For this review, take the finished solid that the model builds, in its own axes (mm). Face numbers are marked on the shaded views. A direction names the side the tool comes from. Round coordinates to 2 decimals unless told otherwise and drop trailing zeros. Loops run counter-clockwise (first coordinate to the right, second up) from the corner with the lowest first, then second, coordinate; pieces in that order, holes last. Notation, with made-up numbers: (77, 63.25) -> (136, 63.25) arc R25 ccw to (136, 77.25) -> close; hole circle Ø9 at (-39.5, 86.25). An arc over 180 degrees is marked (long way). One line per question, with ' | ' between items. Start each with the question number.
1. For pin 1 Ø3 at (y, z) = (-17.5, -16.5) entering from +X; pin 2 Ø2 at (x, y) = (-32, -4.5) entering from -Z; pin 3 Ø2.5 at (x, y) = (-31, -20) entering from -Z, all flat-tipped, find the tip position at first contact; note any pin that passes through.
2. Consider section A-A (y = -23.5). Write out the cut boundary in (x, z), and give its area (3 significant figures).
3. Consider section B-B (x = -27.5). Count the separate pieces of the cut face and the enclosed holes in it, and give its area (3 significant figures).
4. Wall thickness on line 1 along Z through (x, y) = (-25, -9); line 2 along Z through (x, y) = (-19, -36); line 3 along X through (y, z) = (-17, 35): over which ranges is each line inside the solid? List them lowest first.
5. For the marked faces 1, 2 and 3, list the 3-axis set-ups (+Z, -Z, +X, -X, +Y, -Y) from which the entire face can be reached by the end or side of a thin tool; tool diameter is ignored.
6. Draft analysis for pull direction Z (two halves, no side actions). For the marked faces 4, 5 and 6, state which applies: pulls with the +Z half, pulls with the -Z half, needs draft (parallel to the pull), parting line crosses it, or undercut.
```python
from build123d import *

# Parameters (mm, degrees)
F1_DEPTH = 12.7
F2_DEPTH = 25.4
F3_R     = 5.08


with BuildPart() as f1:
    # F0 (on Front) → F1 (new body)
    with BuildSketch(Plane.XZ):
        Polygon((-29.3797869235, -7.2736367583), (-29.3797869235, -44.0696775913), (14.8325152695, -44.0696775913), (15.1177551597, -3.8507485297), (-5.1343315281, 28.666684404), (-5.1343315281, 42.6434762776), (9.1277007014, 42.6434762776), (3.1376483385, 52.341658622), (-34.2288762331, 52.341658622), (-34.2288762331, 46.6368459165), (-25.9568989277, 46.6368459165), (-39.0779674053, 25.529038161), (-39.0779674053, 16.6865773499), (-33.0879166722, 22.1061483026), (-23.674974218, 38.6501066387), (-17.3996798694, 24.958556518), (-17.3996798694, 9.8408022895), align=None)
    extrude(amount=F1_DEPTH)

    # F0 (on Front) + F1_face (on face) + F1_face1 (on face) → F2 (join)
    with BuildSketch(Plane.XZ):
        Polygon((-29.3797869235, -7.2736367583), (-29.3797869235, -44.0696775913), (14.8325152695, -44.0696775913), (15.1177551597, -3.8507485297), (-5.1343315281, 28.666684404), (-5.1343315281, 42.6434762776), (9.1277007014, 42.6434762776), (3.1376483385, 52.341658622), (-34.2288762331, 52.341658622), (-34.2288762331, 46.6368459165), (-25.9568989277, 46.6368459165), (-39.0779674053, 25.529038161), (-39.0779674053, 16.6865773499), (-33.0879166722, 22.1061483026), (-23.674974218, 38.6501066387), (-17.3996798694, 24.958556518), (-17.3996798694, 9.8408022895), align=None)
    with BuildSketch(Plane(origin=(-9.327897656, -12.7, -1.3317405801), x_dir=(1, 0, 0), z_dir=(0, -1, 0))):
        Polygon((18.4555983573, 43.9752168577), (12.4655459944, 53.6733992022), (-24.9009785771, 53.6733992022), (-24.9009785771, 47.9685864966), (-16.6290012717, 47.9685864966), (-29.7500697493, 26.8607787412), (-29.7500697493, 18.01831793), (-23.7600190162, 23.4378888827), (-14.347076562, 39.9818472188), (-8.0717822134, 26.2902970981), (-8.0717822134, 11.1725428697), (-20.0518892675, -5.9418961782), (-20.0518892675, -42.7379370112), (24.1604129255, -42.7379370112), (24.4456528157, -2.5190079495), (4.1935661279, 29.9984249842), (4.1935661279, 43.9752168577), align=None)
    with BuildSketch(Plane(origin=(-9.327897656, 0, -1.3317405801), x_dir=(1, 0, 0), z_dir=(0, 1, 0))):
        Polygon((12.4655459944, -53.6733992022), (18.4555983573, -43.9752168577), (4.1935661279, -43.9752168577), (4.1935661279, -29.9984249842), (24.4456528157, 2.5190079495), (24.1604129255, 42.7379370112), (-20.0518892675, 42.7379370112), (-20.0518892675, 5.9418961782), (-8.0717822134, -11.1725428697), (-8.0717822134, -26.2902970981), (-14.347076562, -39.9818472188), (-23.7600190162, -23.4378888827), (-29.7500697493, -18.01831793), (-29.7500697493, -26.8607787412), (-16.6290012717, -47.9685864966), (-24.9009785771, -47.9685864966), (-24.9009785771, -53.6733992022), align=None)
    extrude(amount=F2_DEPTH, dir=(0, -1, 0))

    # F3
    f3_edges = [f1.edges().sort_by_distance(p)[0] for p in [
        (-39.077967, -38.1, 21.107808),
        (-36.082942, 0, 19.396363),
        (6.132675, -38.1, 47.492567),
        (4.991712, -38.1, 12.407968),
        (-5.134332, -38.1, 35.65508),
        (14.975135, -38.1, -23.960213),
        (-34.228876, -38.1, 49.489252),
        (-23.389733, -38.1, 1.283583),
        (-29.379787, -38.1, -25.671657),
        (-7.273636, -38.1, -44.069678),
    ]]
    fillet(f3_edges, radius=F3_R)


solid = f1.part
```
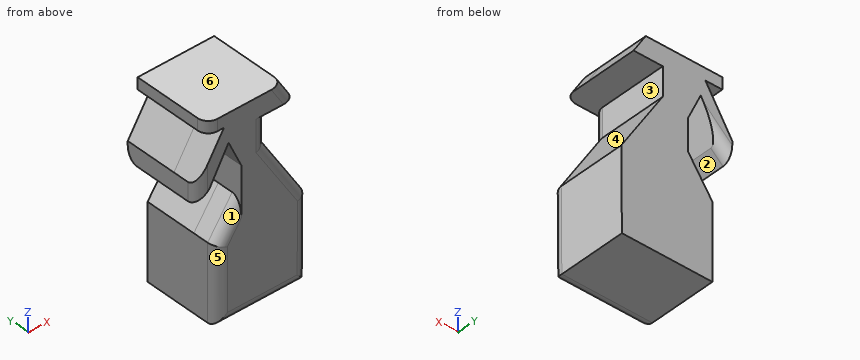
Answer block:
1) pin 1: stops at x = 15.04 | pin 2: stops at z = 22.26 | pin 3: stops at z = 23.58
2) outline: (-39.08, 16.69) -> (-33.09, 22.11) -> (-23.67, 38.65) -> (-17.4, 24.96) -> (-17.4, 9.84) -> (-29.38, -7.27) -> (-29.38, -44.07) -> (14.83, -44.07) -> (15.12, -3.85) -> (-5.13, 28.67) -> (-5.13, 42.64) -> (9.13, 42.64) -> (3.14, 52.34) -> (-34.23, 52.34) -> (-34.23, 46.64) -> (-25.96, 46.64) -> (-39.08, 25.53) -> close | area: 3,340 mm2
3) separate pieces: 3 | enclosed holes: 0 | area: 2,140 mm2
4) line 1: z = -44.07 to -1.02, 36.32 to 52.34 | line 2: z = -43.1 to 5.87, 28.45 to 52.34 | line 3: x = -33.19 to -25.75, -22 to -5.13
5) face 1: -X, -Y | face 2: -Z, +Y, -Y | face 3: +X, +Y, -Y
6) face 4: undercut | face 5: needs draft | face 6: pulls with the +Z half
